```python
from build123d import *

# Parameters (mm, degrees)
SKIZZE1_R                       = 4.57
AUFSATZ_LINEAR_AUSTRAGEN1_DEPTH = 31
SCHNITT_LINEAR_AUSTRAGEN1_DEPTH = 32.666540702
VERRUNDUNG1_R                   = 0.5
KREISMUSTER1_COUNT              = 10
VERRUNDUNG1_OF_KREISMUSTER1_R   = 0.5
FASE1_SIZE                      = 0.2


with BuildPart() as part:
    # Skizze1 → Aufsatz-Linear austragen1 (new body)
    with BuildSketch(Plane(origin=(0, 0, 0), x_dir=(1, 0, 0), z_dir=(0, 1, 0))):
        with Locations(Location((0, 0, 0), (0, 0, 270))):
            Circle(SKIZZE1_R)
    extrude(amount=AUFSATZ_LINEAR_AUSTRAGEN1_DEPTH)

    # Skizze12 → Schnitt-Linear austragen1 (cut, through all)
    with BuildSketch(Plane(origin=(0, 31, 0), x_dir=(1, 0, 0), z_dir=(0, 1, 0))):
        with BuildLine():
            Line((-1.2, 4.409637173), (-0.808470756, 3.57))
            Line((-0.808470756, 3.57), (0.808470756, 3.57))
            Line((0.808470756, 3.57), (1.2, 4.409637173))
            ThreePointArc((1.2, 4.409637173), (0, 4.57), (-1.2, 4.409637173))
        make_face()
    schnitt_linear_austragen1 = extrude(amount=-SCHNITT_LINEAR_AUSTRAGEN1_DEPTH, mode=Mode.SUBTRACT)

    # Verrundung1
    verrundung1_edges = [part.edges().sort_by_distance(p)[0] for p in [
        (0.808470756, 15.5, -3.57),
        (-0.808470756, 15.5, -3.57),
    ]]
    fillet(verrundung1_edges, radius=VERRUNDUNG1_R)

    # Kreismuster1: Schnitt-Linear austragen1 ×10 about axis
    kreismuster1_axis = Axis((0, 0, 0), (0, 1, 0))
    for i in range(1, KREISMUSTER1_COUNT):
        add(schnitt_linear_austragen1.rotate(kreismuster1_axis, i * 360 / KREISMUSTER1_COUNT), mode=Mode.SUBTRACT)

    # Verrundung1 of Kreismuster1
    verrundung1_of_kreismuster1_edges = [part.edges().sort_by_distance(p)[0] for p in [
        (-1.44432677, 15.5, -3.363397857),
        (-2.752459932, 15.5, -2.412983483),
        (-3.14544056, 15.5, -1.872092051),
        (-3.645102966, 15.5, -0.334289289),
        (-3.645102966, 15.5, 0.334289289),
        (-3.14544056, 15.5, 1.872092051),
        (-2.752459932, 15.5, 2.412983483),
        (-1.44432677, 15.5, 3.363397857),
        (-0.808470756, 15.5, 3.57),
        (0.808470756, 15.5, 3.57),
        (1.44432677, 15.5, 3.363397857),
        (2.752459932, 15.5, 2.412983483),
        (3.14544056, 15.5, 1.872092051),
        (3.645102966, 15.5, 0.334289289),
        (3.645102966, 15.5, -0.334289289),
        (3.14544056, 15.5, -1.872092051),
        (2.752459932, 15.5, -2.412983483),
        (1.44432677, 15.5, -3.363397857),
    ]]
    fillet(verrundung1_of_kreismuster1_edges, radius=VERRUNDUNG1_OF_KREISMUSTER1_R)

    # Skizze13 → Schnitt-Rotation1 (revolve, cut)
    with BuildSketch(Plane(origin=(0, 0, 0), x_dir=(0, 0, -1), z_dir=(1, 0, 0)), mode=Mode.PRIVATE) as schnitt_rotation1_sk:
        Polygon((-1.995, 0), (-10.076763041, 0), (-10.076763041, 31), (-1.995, 31), (-1.995, 29), (-2.75, 29), (-2.75, 28.5), (-6.450923694, 28.5), (-6.450923694, 2.5), (-2.75, 2.5), (-2.75, 2), (-1.995, 2), align=None)
    revolve(schnitt_rotation1_sk.sketch.rotate(Axis((0, -5.607699778, 0), (0, 1, 0)), 180), axis=Axis((0, -5.607699778, 0), (0, 1, 0)), mode=Mode.SUBTRACT)

    # Fase1
    fase1_edges = [part.edges().sort_by_distance(p)[0] for p in [
        (0, 31, 1.995),
        (0, 0, 1.995),
        (0, 2, 2.75),
        (0, 29, 2.75),
    ]]
    chamfer(fase1_edges, length=FASE1_SIZE)

    # Skizze14 → Schnitt-Rotation2 (revolve, cut)
    with BuildSketch(Plane(origin=(0, 0, 0), x_dir=(0, 0, -1), z_dir=(1, 0, 0))):
        Polygon((0, 0), (-0.6, 0), (-0.6, 1.5), (0, 1.748528137), align=None)
    revolve(axis=Axis((0, -2.816169131, 0), (0, 1, 0)), mode=Mode.SUBTRACT)


solid = part.part
```
Model file for the job. Use its own axes, mm. A direction names the side the tool comes from. Coordinates: 2 decimals unless noted, no trailing zeros. Use a Markdown table: item, result. Add a question column.
Item 1: Two-plate mould, pull along Z, no slides. Class faces 1 (the face through (0, 16, 3.57)), 2 (the face through (-0.018, 1.736, -0.023)), 3 (the face through (-0.599, 1.087, -1.903)), 4 (the face through (0, 31, 0)): pulls with the +Z half, pulls with the -Z half, needs draft (parallel to the pull), parting line crosses it, or undercut.
Item 2: 3-axis set-ups, long thin cutter, end or side, ignore diameter. For faces 5 (the face through (1, 2, 2)), 6 (the face through (3.397, 15.682, 1.097)), 7 (the face through (-3.397, 15.682, -1.097)), 8 (the face through (-0.599, 29.887, -1.903)): which of +Z, -Z, +X, -X, +Y, -Y reach the whole face in a straight line?
Item 3: Drop flat-ended pins along their axis: pin 1 (0.5 mm diameter, centred on x = 0, y = 10, fed in from -Z); pin 2 (4 mm diameter, centred on x = -1.5, z = 0.5, fed in from -Y); pin 3 (0.8 mm diameter, centred on x = 0, y = 10.5, fed in from +Z); pin 4 (1.5 mm diameter, centred on y = 26, z = 3, fed in from -X). Give the stop position or say it passes through.
Item 4: Drill centre lines: line 1 along Z through (x, y) = (3.75, 24.5); line 2 along Y through (x, z) = (-3.5, 2.25); line 3 along X through (y, z) = (0.5, 0) (3 decimals). Where is each one in solid material? Low to high.
A:
| question | item | result |
|---|---|---|
| 1 | face 1 | pulls with the +Z half |
| 1 | face 2 | undercut |
| 1 | face 3 | parting line crosses it |
| 1 | face 4 | needs draft |
| 2 | face 5 | -Y |
| 2 | face 6 | +X, +Y, -Y |
| 2 | face 7 | -X, +Y, -Y |
| 2 | face 8 | +Y |
| 3 | pin 1 | stops at z = -3.57 |
| 3 | pin 2 | stops at y = 0 |
| 3 | pin 3 | stops at z = 3.57 |
| 3 | pin 4 | stops at x = -3.82 |
| 4 | line 1 | z = -2.61 to -2.44, -0.37 to 0.37, 2.44 to 2.61 |
| 4 | line 2 | y = 2.5 to 28.5 |
| 4 | line 3 | x = -1.995 to -0.6, 0.6 to 1.995 |
